from build123d import *

# Parameters (mm, degrees)
F1_DEPTH = 10
F2_W     = 3.763588
F2_H     = 1.505818
F3_DEPTH = 3
F4_W     = 4.596189
F4_H     = 1.838945
F5_DEPTH = 3


with BuildPart() as f1:
    # F0 (on Front) → F1 (new body)
    with BuildSketch(Plane.XZ):
        Polygon((0, 50.5), (0, 0), (6.841576, 0), (6.841576, 18.445263), (16.01394, 0), (25.11394, 0), align=None)
    extrude(amount=F1_DEPTH)

    # F2 (on face) → F3 (join)
    with BuildSketch(Plane(origin=(0, 0, 0), x_dir=(1, 0, 0), z_dir=(0, 0, -1))):
        with Locations((3.376952, 5.229204)):
            Rectangle(F2_W, F2_H)
    extrude(amount=F3_DEPTH)

    # F4 (on face) → F5 (join)
    with BuildSketch(Plane(origin=(0, 0, 0), x_dir=(1, 0, 0), z_dir=(0, 0, -1))):
        with Locations((20.651922, 5.366659)):
            Rectangle(F4_W, F4_H)
    extrude(amount=F5_DEPTH)


solid = f1.part
Design review of the part built by this model. Coordinates are the model's own, in mm. A direction names the side the tool comes from. Round coordinates to 2 decimals unless told otherwise and drop trailing zeros. Write each loop counter-clockwise with the first axis right and the second up, starting at its lowest first coordinate (ties: lowest second). Pieces come first, ordered by that corner, then holes. Notation, with made-up numbers: M -25,7 L -3,7 A29 ccw -3,40 Z; hole C 4,17 d2. An arc over 180 degrees is marked long. One line per item, written item: value. Start each with the question number.
1. Clearance check with flat-ended pins moving along their axes: P1, Ø0.9, axis at x = 3.5, z = -1.5, coming from the -Y side; P2, Ø3.5, axis at x = 4, z = -2, coming from the +Y side; P3, Ø3, axis at y = -6.5, z = 7.5, coming from the +X side. State where each tip first meets the part, or that it passes through.
2. Take a section at B-B on z = 15. State the section outline as (x, y) points.
3. Draft analysis for pull direction X (two halves, no side actions). For faces 1 (the face through (6.842, -5, 9)), 2 (the face through (21, -5, -3)), 3 (the face through (12.73, -4.93, 24.9)), state which applies: pulls with the +X half, pulls with the -X half, needs draft (parallel to the pull), parting line crosses it, or undercut.
4. Take a section at C-C on x = 19.75. State the section outline as (y, z) points.
5. For faces 4 (the face through (21, -6.286, -1)), 5 (the face through (3, -5.982, -1)), 6 (the face through (1.495, -5, -1)), list the 3-axis set-ups (+Z, -Z, +X, -X, +Y, -Y) from which the entire face can be reached by the end or side of a thin tool; tool diameter is ignored.
6. Take a section at A-A on y = -2.5. State the section outline as (x, z) points.
7. To check wall thickness, follow probe 1 along X at (y, z) = (-5, 13); probe 2 along X at (y, z) = (-7.25, 10.5); probe 3 along Z at (x, y) = (8, -3.5). State the ranges of each line that lie inside material, in increasing order. Write a range as from..to.
8. Take a section at D-D on y = -5. State the section outline as (x, z) points, then the cut area to 3 significant figures.
Computed:
1. P1: stops at y = -5.98
1. P2: stops at y = -4.48
1. P3: stops at x = 22.13
2. outline: M 0,-10 L 6.84,-10 L 6.84,0 L 0,0 Z; M 8.55,-10 L 17.65,-10 L 17.65,0 L 8.55,0 Z
3. face 1: undercut
3. face 2: needs draft
3. face 3: pulls with the +X half
4. outline: M -10,0 L -6.29,0 L -6.29,-3 L -4.45,-3 L -4.45,0 L 0,0 L 0,10.79 L -10,10.79 Z
5. face 4: -Z, +X, -X, -Y
5. face 5: -Z, -X, -Y
5. face 6: -Z, -X, +Y, -Y
6. outline: M 0,0 L 6.84,0 L 6.84,18.45 L 16.01,0 L 25.11,0 L 0,50.5 Z
7. probe 1: x = 0..6.84, 9.55..18.65
7. probe 2: x = 0..6.84, 10.79..19.89
7. probe 3: z = 16.12..34.41
8. outline: M 0,0 L 1.5,0 L 1.5,-3 L 5.26,-3 L 5.26,0 L 6.84,0 L 6.84,18.45 L 16.01,0 L 18.35,0 L 18.35,-3 L 22.95,-3 L 22.95,0 L 25.11,0 L 0,50.5 Z
8. area: 575 mm²
